from build123d import *

# Parameters (mm, degrees)
SKETCH2_W           = 238
SKETCH2_H           = 165
BOSS_EXTRUDE1_DEPTH = 4
SKETCH3_W           = 4
SKETCH3_H           = 30
CUT_EXTRUDE1_DEPTH  = 290.629073126
SKETCH5_R           = 45.261498606
CUT_EXTRUDE3_DEPTH  = 10
SKETCH8_W           = 45
SKETCH8_H           = 25
CUT_EXTRUDE4_DEPTH  = 290.629073126


with BuildPart() as part:
    # Sketch2 → Boss-Extrude1 (new body)
    with BuildSketch(Plane(origin=(0, 0, 0), x_dir=(1, 0, 0), z_dir=(0, 1, 0))):
        with Locations((119, 82.5)):
            Rectangle(SKETCH2_W, SKETCH2_H)
    extrude(amount=BOSS_EXTRUDE1_DEPTH)

    # Sketch3 → Cut-Extrude1 (cut, through all)
    with BuildSketch(Plane(origin=(0, 4, 0), x_dir=(1, 0, 0), z_dir=(0, 1, 0))):
        with Locations((226, 101.931901068)):
            Rectangle(SKETCH3_W, SKETCH3_H)
        with Locations((226, 41.931901068)):
            Rectangle(SKETCH3_W, SKETCH3_H)
        with Locations((12, 101.931901068)):
            Rectangle(SKETCH3_W, SKETCH3_H)
        with Locations((12, 41.931901068)):
            Rectangle(SKETCH3_W, SKETCH3_H)
    extrude(amount=-CUT_EXTRUDE1_DEPTH, mode=Mode.SUBTRACT)

    # Sketch5 → Cut-Extrude3 (cut)
    with BuildSketch(Plane(origin=(0, 4, 0), x_dir=(1, 0, 0), z_dir=(0, 1, 0))):
        with Locations((238, 165)):
            Circle(SKETCH5_R)
        with Locations((0, 165)):
            Circle(SKETCH5_R)
    extrude(amount=-CUT_EXTRUDE3_DEPTH, mode=Mode.SUBTRACT)

    # Sketch8 → Cut-Extrude4 (cut, through all)
    with BuildSketch(Plane(origin=(0, 4, 0), x_dir=(1, 0, 0), z_dir=(0, 1, 0))):
        with Locations((76.5, 42.5)):
            Rectangle(SKETCH8_W, SKETCH8_H)
        with Locations((161.5, 42.5)):
            Rectangle(SKETCH8_W, SKETCH8_H)
    extrude(amount=-CUT_EXTRUDE4_DEPTH, mode=Mode.SUBTRACT)


solid = part.part
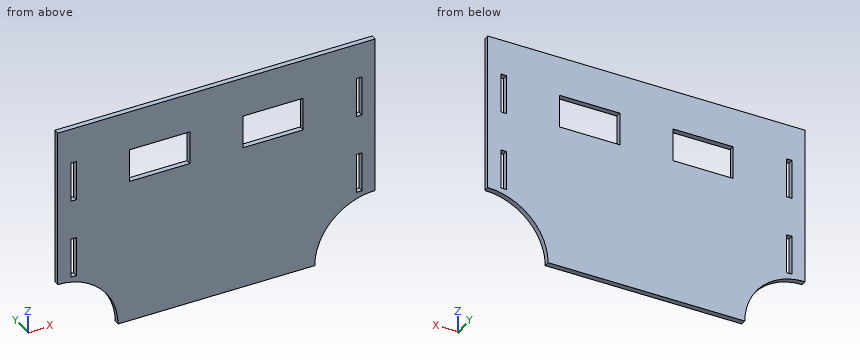
Part model, mm, in its own coordinate system. Round coordinates to 2 decimals unless told otherwise and drop trailing zeros. Write each loop counter-clockwise with the first axis right and the second up, starting at its lowest first coordinate (ties: lowest second). Pieces come first, ordered by that corner, then holes. Notation, with made-up numbers: M 83,-23.5 L 129,-23.5 A30 cw 129,12.5 Z; hole C 20.5,53 d6. An arc over 180 degrees is marked long. Return JSON: item names as keys, results as strings. Group by question number.
(1) Saw through at A-A on z = -44. Write the cut outline in (x, y).
(2) Saw through at D-D on z = -109. Write the cut outline in (x, y).
(3) Pin check, flat tips, straight feed: pin 1 Ø1.2 at (x, y) = (11, 2.5) entering from -Z; pin 2 Ø2 at (x, y) = (203, 2) entering from -Z. Stop position of each tip, or through.
(4) Saw through at B-B on x = 94. Write the cut outline in (y, z).
(5) Saw through at C-C on y = 1.2. Count the separate pieces of the cut face and the enclosed holes in it, then the cut area to 3 significant figures.
(6) Drill centre lines: probe 1 along X at (y, z) = (0.25, -107.5); probe 2 along X at (y, z) = (0.55, -47.5); probe 3 along Z at (x, y) = (155, 3.25). Where is each one in solid material? Low to high.
Returned:
{
 "1": {"outline": "M 0,0 L 10,0 L 10,4 L 0,4 Z; M 14,0 L 54,0 L 54,4 L 14,4 Z; M 99,0 L 139,0 L 139,4 L 99,4 Z; M 184,0 L 224,0 L 224,4 L 184,4 Z; M 228,0 L 238,0 L 238,4 L 228,4 Z"},
 "2": {"outline": "M 0,0 L 10,0 L 10,4 L 0,4 Z; M 14,0 L 224,0 L 224,4 L 14,4 Z; M 228,0 L 238,0 L 238,4 L 228,4 Z"},
 "3": {"pin 1": "z = -121.25", "pin 2": "z = -137.57"},
 "4": {"outline": "M 0,-165 L 4,-165 L 4,-55 L 0,-55 Z; M 0,-30 L 4,-30 L 4,0 L 0,0 Z"},
 "5": {"separate pieces": "1", "enclosed holes": "6", "area": "33,300 mm²"},
 "6": {"probe 1": "0 to 10, 14 to 224, 228 to 238", "probe 2": "0 to 10, 14 to 54, 99 to 139, 184 to 224, 228 to 238", "probe 3": "-165 to -55, -30 to 0"}
}
